The listing builds one solid part. Answer for the finished solid, in the listing's coordinates (mm). Face numbers are marked on the shaded views. A direction names the side the tool comes from. Coordinates: 2 decimals unless noted, no trailing zeros. Order: outer loops, then holes, each group sorted by start corner. A loop starts at its lowest first (then second) coordinate and runs counter-clockwise, first axis right, second up.
from build123d import *

# Parameters (mm, degrees)
SKETCH1_R           = 1.75
BOSS_EXTRUDE1_DEPTH = 1.9
SKETCH2_W           = 28.5
SKETCH2_H           = 54.8
BOSS_EXTRUDE2_DEPTH = 0.9
CHAMFER1_SIZE       = 1
BOSS_EXTRUDE3_DEPTH = 19
CUT_EXTRUDE1_DEPTH  = 18.3
SKETCH5_W           = 3.5
SKETCH5_H           = 3.5
SKETCH5_W_2         = 3.4
SKETCH5_H_2         = 3.4
SKETCH5_W_3         = 7
SKETCH5_H_3         = 0.05
SKETCH5_W_4         = 21
SKETCH5_H_4         = 15
SKETCH5_W_5         = 20.9
SKETCH5_H_5         = 14.9
CUT_EXTRUDE2_DEPTH  = 0.05
SKETCH6_W           = 24
SKETCH6_H           = 15.5
CUT_EXTRUDE3_DEPTH  = 19
CUT_EXTRUDE4_DEPTH  = 1.25
SKETCH8_W           = 20
SKETCH8_H           = 13
BOSS_EXTRUDE4_DEPTH = 14
SKETCH5_3_W         = 16
SKETCH5_3_H         = 10.5
CUT_EXTRUDE6_DEPTH  = 1
SKETCH10_W          = 7.9
SKETCH10_H          = 10.3
REVOLVE2_ANGLE      = 30
SKETCH10_6_W        = 7.9
SKETCH10_6_H        = 10.3
REVOLVE3_ANGLE      = 15
FILLET1_R           = 18


with BuildPart() as part:
    # Sketch1 → Boss-Extrude1 (new body)
    with BuildSketch(Plane.XY):
        Polygon((-24.5, 0), (-14, 29.5), (14, 29.5), (24.5, 0), (14, -29.5), (-14, -29.5), align=None)
        with Locations((-19.85, 0)):
            Circle(SKETCH1_R, mode=Mode.SUBTRACT)
        with Locations((19.85, 0)):
            Circle(SKETCH1_R, mode=Mode.SUBTRACT)
    extrude(amount=BOSS_EXTRUDE1_DEPTH)

    # Sketch2 → Boss-Extrude2 (add)
    with BuildSketch(Plane.XY.offset(1.9)):
        Rectangle(SKETCH2_W, SKETCH2_H)
    extrude(amount=BOSS_EXTRUDE2_DEPTH)

    # Chamfer1
    chamfer1_edges = [part.edges().sort_by_distance(p)[0] for p in [
        (-21.6, 0, 1.9),
        (18.1, 0, 1.9),
    ]]
    chamfer(chamfer1_edges, length=CHAMFER1_SIZE)

    # Sketch3 → Boss-Extrude3 (add)
    with BuildSketch(Plane(origin=(0, 0, 0), x_dir=(-1, 0, 0), z_dir=(0, 0, -1))):
        Polygon((7.5, 24.6), (-7.5, 24.6), (-13.5, 18.65), (-13.5, -22.5), (13.5, -22.5), (13.5, 18.65), align=None)
    extrude(amount=BOSS_EXTRUDE3_DEPTH)

    # Sketch4 → Cut-Extrude1 (cut)
    with BuildSketch(Plane.XY.offset(2.8)):
        Polygon((7.5, 23.25), (-7.5, 23.25), (-12, 18.65), (-12, 6.65), (12, 6.65), (12, 18.65), align=None)
    extrude(amount=-CUT_EXTRUDE1_DEPTH, mode=Mode.SUBTRACT)

    # Sketch5 → Cut-Extrude2 (cut)
    with BuildSketch(Plane.XY.offset(2.8)):
        with Locations((-5.25, 0.95)):
            Rectangle(SKETCH5_W, SKETCH5_H)
        with Locations((-5.25, 0.95)):
            Rectangle(SKETCH5_W_2, SKETCH5_H_2, mode=Mode.SUBTRACT)
        Polygon((-3.5, 2.05), (0, 2.05), (3.5, 2.05), (3.5, 2.1), (0, 2.1), (-3.5, 2.1), align=None)
        with Locations((0, -0.175)):
            Rectangle(SKETCH5_W_3, SKETCH5_H_3)
        with Locations((5.25, 0.95)):
            Rectangle(SKETCH5_W, SKETCH5_H)
        with Locations((5.25, 0.95)):
            Rectangle(SKETCH5_W_2, SKETCH5_H_2, mode=Mode.SUBTRACT)
        with Locations((0, -13.7)):
            Rectangle(SKETCH5_W_4, SKETCH5_H_4)
        with Locations((0, -13.7)):
            Rectangle(SKETCH5_W_5, SKETCH5_H_5, mode=Mode.SUBTRACT)
        Polygon((-4.5, 6.65), (-4.5, 5.15), (-11.75, 5.15), (-11.75, -3.25), (11.75, -3.25), (11.75, 5.15), (4.5, 5.15), (4.5, 6.65), (4.55, 6.65), (4.55, 5.2), (11.8, 5.2), (11.8, -3.3), (-11.8, -3.3), (-11.8, 5.2), (-4.55, 5.2), (-4.55, 6.65), align=None)
    extrude(amount=-CUT_EXTRUDE2_DEPTH, mode=Mode.SUBTRACT)

    # Sketch6 → Cut-Extrude3 (cut)
    with BuildSketch(Plane(origin=(0, 0, -19), x_dir=(-1, 0, 0), z_dir=(0, 0, -1))):
        with Locations((0, -13.5)):
            Rectangle(SKETCH6_W, SKETCH6_H)
    extrude(amount=-CUT_EXTRUDE3_DEPTH, mode=Mode.SUBTRACT)

    # Sketch7 → Cut-Extrude4 (cut)
    with BuildSketch(Plane.XZ.offset(22.5)):
        Polygon((8.5, -19), (4.458548116, -12), (-4.458548116, -12), (-8.5, -19), align=None)
    extrude(amount=-CUT_EXTRUDE4_DEPTH, mode=Mode.SUBTRACT)

    # Sketch8 → Boss-Extrude4 (add)
    with BuildSketch(Plane(origin=(0, 0, 0), x_dir=(-1, 0, 0), z_dir=(0, 0, -1))):
        with Locations((0, -13.5)):
            Rectangle(SKETCH8_W, SKETCH8_H)
    extrude(amount=BOSS_EXTRUDE4_DEPTH)

    # Sketch5<3> → Cut-Extrude6 (cut)
    with BuildSketch(Plane.XY.offset(2.8)):
        with Locations((0, -13.7)):
            Rectangle(SKETCH5_3_W, SKETCH5_3_H)
    extrude(amount=-CUT_EXTRUDE6_DEPTH, mode=Mode.SUBTRACT)

    # Sketch10 → Revolve2 (revolve)
    with BuildSketch(Plane.XY.offset(1.8)):
        with Locations((-3.95, -13.7)):
            Rectangle(SKETCH10_W, SKETCH10_H)
    revolve(axis=Axis((0, -8.45, 1.8), (0, 1, 0)), revolution_arc=REVOLVE2_ANGLE)

    # Sketch10<6> → Revolve3 (revolve)
    with BuildSketch(Plane.XY.offset(1.8)):
        with Locations((3.95, -13.7)):
            Rectangle(SKETCH10_6_W, SKETCH10_6_H)
    revolve(axis=Axis((0, -8.45, 1.8), (0, -1, 0)), revolution_arc=REVOLVE3_ANGLE)

    # Fillet1
    fillet1_edges = [part.edges().sort_by_distance(p)[0] for p in [
        (0, -13.7, 1.8),
    ]]
    fillet(fillet1_edges, radius=FILLET1_R)


solid = part.part
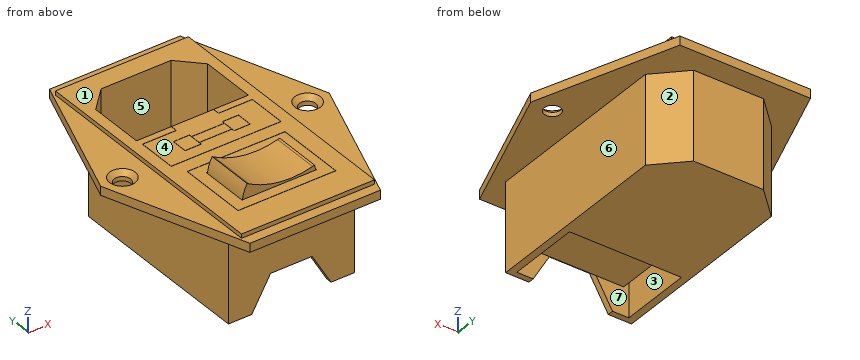
(1) A tool of negligible diameter and unlimited length cuts with its end or side. For the marked faces 4, 5, 6 and 7, from which of +Z, -Z, +X, -X, +Y, -Y can it reach the whole face along a straight path? Write none if from no direction.
(2) Given pin 1 Ø1 at (y, z) = (-5.5, -8.5) entering from +X; pin 2 Ø5 at (x, y) = (11.5, 23.5) entering from +Z; pin 3 Ø3 at (x, y) = (-2, -13) entering from +Z, each flat-ended and moving along its own axis, determine where each tip first touches the part or whether it passes through.
(3) Find section B-B on y = 7.5. Determine the outline of the cut face in (x, z), then the cut area to 3 significant figures.
(4) The mould has two halves that part along Y. Classify the marked faces 1, 2 and 3: pulls with the +Y half, pulls with the -Y half, needs draft (parallel to the pull), parting line crosses it, or undercut.
(5) Find the intervals of material crossed by probe 1 along Y at (x, z) = (2.5, -13.25); probe 2 along X at (y, z) = (12, -3); probe 3 along Z at (x, y) = (-8.5, 6.5), in increasing order.
(6) Find section A-A on x = 19.85. Determine the outline of the cut face in (y, z), then the cut area to 3 significant figures.
(7) Find section C-C on y = -5. Determine the outline of the cut face in (x, z), then the cut area to 3 significant figures.
Resolved:
1. face 4: +Z, +X, -X, +Y
1. face 5: +Z
1. face 6: -Z, +X, +Y, -Y
1. face 7: -Z
2. pin 1: stops at x = 13.5
2. pin 2: stops at z = 2.8
2. pin 3: stops at z = 4.16
3. outline: (-21.83, 0) - (-13.5, 0) - (-13.5, -19) - (13.5, -19) - (13.5, 0) - (21.83, 0) - (21.83, 1.9) - (14.25, 1.9) - (14.25, 2.8) - (12, 2.8) - (12, -15.5) - (-12, -15.5) - (-12, 2.8) - (-14.25, 2.8) - (-14.25, 1.9) - (-21.83, 1.9) - close
3. area: 182 mm2
4. face 1: needs draft
4. face 2: pulls with the +Y half
4. face 3: undercut
5. probe 1: y = -20 to -7, -5.75 to 6.65, 23.25 to 24.6
5. probe 2: x = -13.5 to -12, 12 to 13.5
5. probe 3: z = -19 to 2.8
6. outline: (-13.06, 0) - (-1.75, 0) - (-1.75, 0.9) - (-2.75, 1.9) - (-13.06, 1.9) - close; (1.75, 0) - (13.06, 0) - (13.06, 1.9) - (2.75, 1.9) - (1.75, 0.9) - close
6. area: 42.0 mm2
7. outline: (-22.72, 0) - (-13.5, 0) - (-13.5, -19) - (13.5, -19) - (13.5, 0) - (22.72, 0) - (22.72, 1.9) - (14.25, 1.9) - (14.25, 2.8) - (-14.25, 2.8) - (-14.25, 1.9) - (-22.72, 1.9) - close
7. area: 625 mm2
